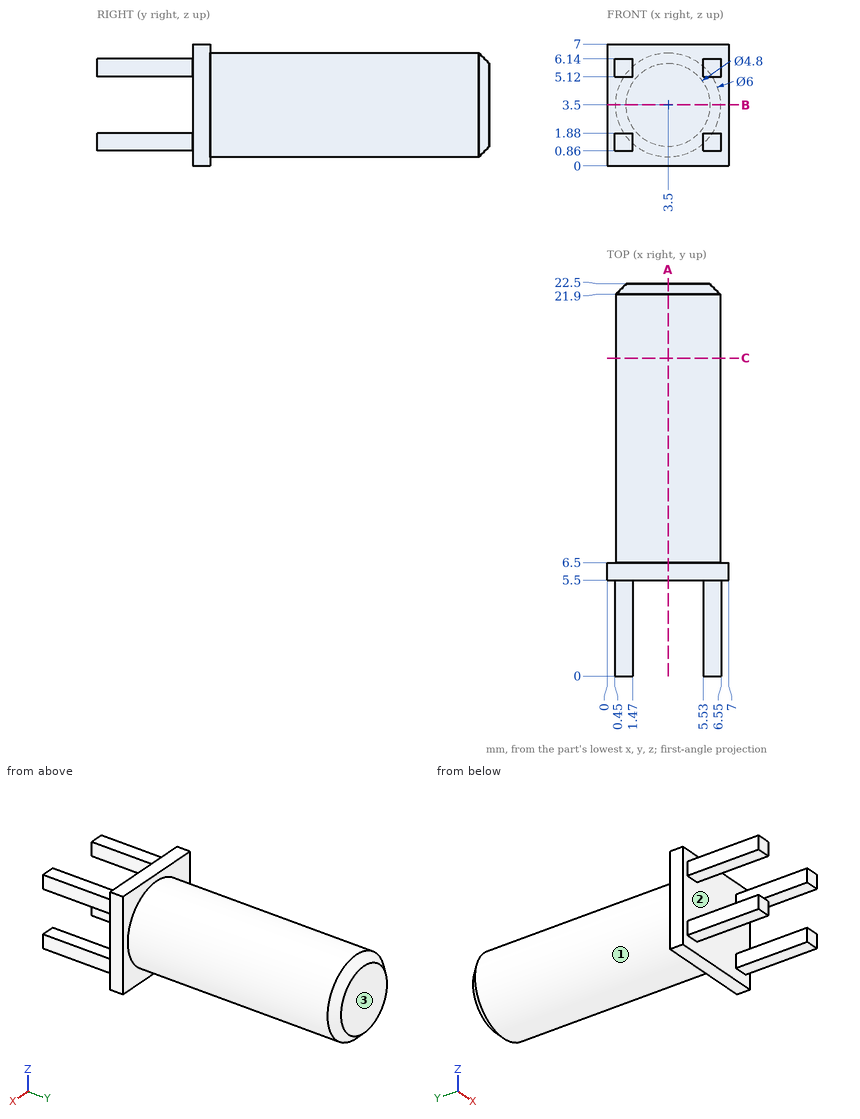
Geometry check sheet. Reference: drawing and pictorial views, mm from the part's lowest x, y, z. Round coordinates to 2 decimals unless told otherwise and drop trailing zeros. Order: outer loops, then holes, each group sorted by start corner. A loop starts at its lowest first (then second) coordinate and runs counter-clockwise, first axis right, second up.
Q1. Cross-section at B-B, the plane z = 3.5. Enter the section's corners in (x, y), plus the area to 3 significant figures.
Filled sheet:
outline: (0, 5.5) - (7, 5.5) - (7, 6.5) - (6.5, 6.5) - (6.5, 21.9) - (5.9, 22.5) - (1.1, 22.5) - (0.5, 21.9) - (0.5, 6.5) - (0, 6.5) - close
area: 103 mm2
Q2. Draft check along X on the marked faces 1, 2 and 3. Enter one of: pulls with the +X half, pulls with the -X half, needs draft (parallel to the pull), parting line crosses it, or undercut.
Filled sheet:
face 1: parting line crosses it
face 2: undercut
face 3: needs draft
Q3. Cross-section at A-A, the plane x = 3.5. Enter the section's corners in (y, z).
Filled sheet:
outline: (5.5, 0) - (6.5, 0) - (6.5, 0.5) - (21.9, 0.5) - (22.5, 1.1) - (22.5, 5.9) - (21.9, 6.5) - (6.5, 6.5) - (6.5, 7) - (5.5, 7) - close
Q4. Depth check by flat-ended pin: P1, Ø2, axis at x = 3, z = 4.5, coming from the -Y side; P2, Ø0.5, axis at y = 3.5, z = 1.5, coming from the +X side; P3, Ø1.1, axis at x = 1, y = 3.5, coming from the +Z side. Enter the tip coordinate at first touch or a pass-through.
Filled sheet:
P1: stops at y = 5.5
P2: stops at x = 6.55
P3: stops at z = 6.14
Q5. Cross-section at C-C, the plane y = 18.25. Enter the section's corners in (x, z).
Filled sheet:
outline: circle Ø6 at (3.5, 3.5)
Q6. Scan lines: L1, parallel to Z at x = 5.75, y = 1.5; L2, parallel to Y at x = 3, z = 2.5; L3, parallel to X at y = 4.5, z = 1.5. Record each from-to range of solid material in increasing order.
Filled sheet:
L1: z = 0.86 to 1.88, 5.12 to 6.14
L2: y = 5.5 to 22.5
L3: x = 0.45 to 1.47, 5.53 to 6.55
